Design review of the part built by this model. Coordinates are the model's own, in mm. A direction names the side the tool comes from. Give positions to 0.01 mm unless a question says otherwise; leave off trailing zeros. Order: outer loops, then holes, each group sorted by start corner. A loop starts at its lowest first (then second) coordinate and runs counter-clockwise, first axis right, second up. Notation, with made-up numbers: M 87,15 L 118,15 A29 cw 118,49 Z; hole C 31,16 d5. An arc over 180 degrees is marked long. Answer as a JSON object with one key per item and string values.
from build123d import *

# Parameters (mm, degrees)
BOSS_EXTRUDE1_DEPTH            = 7.5
BOSS_EXTRUDE2_DEPTH            = 7.5
CUT_EXTRUDE1_DEPTH             = 5
F_3_2_3_2_DIAMETER_HOLE1_D     = 3.2
FILLET1_R                      = 2
FILLET2_R                      = 2
CUT_EXTRUDE2_REACH             = 39.378
CUT_EXTRUDE2_END_RADIUS        = 224.5
SKETCH22_R                     = 2.1
CUT_EXTRUDE2_DIRECTION_2_DEPTH = 0.9
SKETCH23_R                     = 3.5
CUT_EXTRUDE3_DEPTH             = 2.6
SKETCH24_W                     = 2.6
SKETCH24_H                     = 3.5


with BuildPart() as part:
    # Sketch1 → Boss-Extrude1 (new body)
    with BuildSketch(Plane(origin=(0, 0, 0), x_dir=(1, 0, 0), z_dir=(0, 1, 0))):
        with BuildLine():
            ThreePointArc((-207.414551525, 32.851237658), (-210, 0), (-207.414551525, -32.851237658))
            Line((-207.414551525, -32.851237658), (-217.291434931, -34.415582309))
            ThreePointArc((-217.291434931, -34.415582309), (-220, 0), (-217.291434931, 34.415582309))
            Line((-217.291434931, 34.415582309), (-207.414551525, 32.851237658))
        make_face()
        with BuildLine():
            ThreePointArc((-217.291434931, -34.415582309), (-220, 0), (-217.291434931, 34.415582309))
            Line((-217.291434931, 34.415582309), (-220.254499953, 34.884885704))
            ThreePointArc((-220.254499953, 34.884885704), (-223, 0), (-220.254499953, -34.884885704))
            Line((-220.254499953, -34.884885704), (-217.291434931, -34.415582309))
        make_face()
        with BuildLine():
            Line((-204.451486503, 32.381934263), (-207.414551525, 32.851237658))
            ThreePointArc((-207.414551525, 32.851237658), (-210, 0), (-207.414551525, -32.851237658))
            Line((-207.414551525, -32.851237658), (-204.451486503, -32.381934263))
            ThreePointArc((-204.451486503, -32.381934263), (-207, 0), (-204.451486503, 32.381934263))
        make_face()
    extrude(amount=BOSS_EXTRUDE1_DEPTH)

    # Sketch19 → Boss-Extrude2 (add)
    with BuildSketch(Plane(origin=(0, 0, 0), x_dir=(1, 0, 0), z_dir=(0, 1, 0))):
        with BuildLine():
            Line((-224.019328267, 14.683002512), (-222.522539882, 14.584897818))
            ThreePointArc((-222.522539882, 14.584897818), (-223, 0), (-222.522539882, -14.584897818))
            Line((-222.522539882, -14.584897818), (-224.019328267, -14.683002512))
            ThreePointArc((-224.019328267, -14.683002512), (-224.5, 0), (-224.019328267, 14.683002512))
        make_face()
    extrude(amount=BOSS_EXTRUDE2_DEPTH)

    # Sketch15 → Cut-Extrude1 (cut)
    with BuildSketch(Plane(origin=(0, 7.5, 0), x_dir=(1, 0, 0), z_dir=(0, 1, 0))):
        with BuildLine():
            Line((-219.772609758, 10), (-209.761769634, 10))
            ThreePointArc((-209.761769634, 10), (-208.900850883, 21.457737542), (-207.414551525, 32.851237658))
            Line((-207.414551525, 32.851237658), (-217.291434931, 34.415582309))
            ThreePointArc((-217.291434931, 34.415582309), (-218.872736893, 22.242415451), (-219.772609758, 10))
        make_face()
        with BuildLine():
            ThreePointArc((-207.414551525, -32.851237658), (-208.900850883, -21.457737542), (-209.761769634, -10))
            Line((-209.761769634, -10), (-219.772609758, -10))
            ThreePointArc((-219.772609758, -10), (-218.872736893, -22.242415451), (-217.291434931, -34.415582309))
            Line((-217.291434931, -34.415582309), (-207.414551525, -32.851237658))
        make_face()
    extrude(amount=-CUT_EXTRUDE1_DEPTH, mode=Mode.SUBTRACT)

    # Ø3.2 (3.2) Diameter Hole1 (through all)
    with Locations(Plane(origin=(0, 0, 0), x_dir=(-1, 0, 0), z_dir=(0, -1, 0))):
        with Locations((214.18186009, -18.738484691), (214.18186009, 18.738484691)):
            Hole(F_3_2_3_2_DIAMETER_HOLE1_D / 2)

    # Fillet1
    fillet1_edges = [part.edges().sort_by_distance(p)[0] for p in [
        (-220.254499953, 3.75, 34.884885704),
        (-220.254499953, 3.75, -34.884885704),
        (-204.451486503, 3.75, -32.381934263),
        (-204.451486503, 3.75, 32.381934263),
    ]]
    fillet(fillet1_edges, radius=FILLET1_R)

    # Fillet2
    # the kernel refuses this fillet: 2 mm, written as the material it adds along each edge
    with BuildSketch(Plane(origin=(-222.522539882, 0, -14.584897818), x_dir=(0.06970140258603677, 0, -0.9975678996827931), z_dir=(0, 1, 0))) as fillet2_piece_1:
        with BuildLine():
            CenterArc((1.930030715, 1.99998144), FILLET2_R, 194.477374901, 75.275788142)
            Line((-0.006462156, 1.49998608), (-0.045192014, 1.489986173))
            ThreePointArc((-0.045192014, 1.489986173), (-0.043230707, 0.749820716), (-0.039999629, -0.000172324))
            Line((-0.039999629, -0.000172324), (0.000172324, -0.039999629))
            ThreePointArc((0.000172324, -0.039999629), (0.960707253, -0.037930577), (1.921242182, -0.039999629))
            Line((1.921242182, -0.039999629), (1.921414506, 0))
        make_face()
    extrude(amount=7.5)
    with BuildSketch(Plane(origin=(-222.522539882, 0, 14.584897818), x_dir=(-0.9978589232386029, 0, 0.06540312923015226), z_dir=(0, 1, 0))) as fillet2_piece_2:
        with BuildLine():
            CenterArc((1.991648107, 1.938628933), FILLET2_R, 180.493673912, 75.275788142)
            Line((-0.008277654, 1.921396676), (-0.048276169, 1.92105203))
            ThreePointArc((-0.048276169, 1.92105203), (-0.042069052, 0.960534929), (-0.04, 0))
            Line((-0.04, 0), (0, -0.04))
            ThreePointArc((0, -0.04), (0.75, -0.04), (1.490167038, -0.038772579))
            Line((1.490167038, -0.038772579), (1.5, 0))
        make_face()
    extrude(amount=7.5)

    # Cut-Extrude2: up to this cylinder (the profile starts inside it)
    cut_extrude2_end = Plane(origin=(0, 7.5, 0), z_dir=(0, -1, 0)) * Cylinder(CUT_EXTRUDE2_END_RADIUS, 528.756, mode=Mode.PRIVATE)
    # Sketch22 → Cut-Extrude2 (cut, up to the surface)
    with BuildSketch(Plane(origin=(-212.5, 0, 0), x_dir=(0, 0, -1), z_dir=(1, 0, 0)), mode=Mode.PRIVATE) as cut_extrude2_sk1:
        with Locations((0, 7.5)):
            Circle(SKETCH22_R)
    cut_extrude2_tool1 = extrude(cut_extrude2_sk1.sketch, amount=-CUT_EXTRUDE2_REACH, mode=Mode.PRIVATE) & cut_extrude2_end
    add(cut_extrude2_tool1.solids().sort_by_distance((-212.5, 7.5, 0))[0], mode=Mode.SUBTRACT)

    # Sketch22 → Cut-Extrude2 direction 2 (cut)
    with BuildSketch(Plane(origin=(-212.5, 0, 0), x_dir=(0, 0, -1), z_dir=(1, 0, 0))):
        with Locations((0, 7.5)):
            Circle(SKETCH22_R)
    extrude(amount=CUT_EXTRUDE2_DIRECTION_2_DEPTH, mode=Mode.SUBTRACT)

    # Sketch23 → Cut-Extrude3 (cut)
    with BuildSketch(Plane.ZY.offset(211.6)):
        with Locations((0, 7.439199918)):
            Circle(SKETCH23_R)
    extrude(amount=CUT_EXTRUDE3_DEPTH, mode=Mode.SUBTRACT)

    # Sketch24 → Cut-Revolve1 (revolve, cut)
    with BuildSketch(Plane(origin=(0, 7.5, 0), x_dir=(1, 0, 0), z_dir=(0, 1, 0))):
        with Locations((-223.2, 1.75)):
            Rectangle(SKETCH24_W, SKETCH24_H)
    revolve(axis=Axis((-224.5, 7.5, 0), (1, 0, 0)), mode=Mode.SUBTRACT)


solid = part.part
(1) We need section C-C (z = 12.5). Write out the cut boundary in (x, y), plus the area to 3 significant figures.
Checked values:
{"outline": "M -224.15,0 L -206.62,0 L -206.62,7.5 L -209.63,7.5 L -209.63,2.5 L -219.64,2.5 L -219.64,7.5 L -224.15,7.5 Z", "area": "81.4 mm^2"}
(2) Insertion check: pin 1 (1.8 mm diameter, centred on y = 5, z = 1, fed in from -X); pin 2 (1.1 mm diameter, centred on y = 5.5, z = -1.5, fed in from +X); pin 3 (1.5 mm diameter, centred on y = 2, z = 11, fed in from +X); pin 4 (5 mm diameter, centred on x = -214.18, z = -18.74, fed in from +Y). Each pin has a flat end and moves straight along its axis. Give the tip position at first contact, or say it passes through.
Checked values:
{"pin 1": "stops at x = -224.5", "pin 2": "stops at x = -206.99", "pin 3": "stops at x = -206.67", "pin 4": "stops at y = 2.5"}
(3) We need section D-D (z = -28). Write out the cut boundary in (x, y), plus the area to 3 significant figures.
Checked values:
{"outline": "M -221.24,0 L -205.1,0 L -205.1,7.5 L -208.12,7.5 L -208.12,2.5 L -218.21,2.5 L -218.21,7.5 L -221.24,7.5 Z", "area": "70.6 mm^2"}
(4) To check wall thickness, follow L1, parallel to X at y = 7.25, z = -18; L2, parallel to Y at x = -215.25, z = 24; L3, parallel to Z at x = -215.25, y = 6.75. State the ranges of each line that lie inside material, in increasing order. Write a range as from..to.
Checked values:
{"L1": "x = -222.27..-219.26, -209.23..-206.22", "L2": "y = 0..2.5", "L3": "z = -10..-1.96, 1.96..10"}
(5) Tool access review of faces 5 (the flat face through (-221.9, 5, 0)), 6 (the cylindrical face through (-221.614, 3.698, -24.828)), 7 (the flat face through (-215, 5, -10)): name each direction out of +Z, -Z, +X, -X, +Y, -Y from which nothing blocks a thin tool from reaching the whole face with its end or side.
Checked values:
{"face 5": "-X, +Y", "face 6": "-Z, -X, +Y, -Y", "face 7": "+Y"}
(6) We need section A-A (z = 0). Write out the cut boundary in (x, y).
Checked values:
{"outline": "M -224.5,0 L -207,0 L -207,7.5 L -211.6,7.5 L -211.6,3.94 L -214.2,3.94 L -214.2,5.4 L -221.9,5.4 L -221.9,4 L -224.5,4 Z"}
(7) Draft analysis for pull direction Z (two halves, no side actions). For faces 1 (the cylindrical face through (-208.917, 5.035, -21.298)), 2 (the cylindrical face through (-223, 4, 0)), 3 (the cylindrical face through (-215.78, 1.27, 18.67)), 4 (the cylindrical face through (-222.88, 3.7, 15.33)), state which applies: +Z half, -Z half, draft (parallel to the pull), parting line (faces both ways), or undercut.
Checked values:
{"face 1": "-Z half", "face 2": "undercut", "face 3": "undercut", "face 4": "+Z half"}
